Here's how the part is built. I have some questions about the finished solid (model axes, mm). Face numbers are marked on the shaded views. Round coordinates to 2 decimals unless told otherwise and drop trailing zeros. Loops run counter-clockwise (first coordinate to the right, second up) from the corner with the lowest first, then second, coordinate; pieces in that order, holes last. Notation, with made-up numbers: (22, 39) - (51, 39) arc R18 ccw to (51, 74) - close; hole circle Ø5 at (-2.5, -1.5). An arc over 180 degrees is marked (long way). Answer as a JSON object with one key per item and string values. Group by question number.
1) I want a section at A-A, the plane x = 0. Please give me the cut outline in (y, z).
2) If we mould it in two halves opening along Y, with no side actions, what happens to the marked faces 1, 2 and 3? For each: pulls with the +Y half, pulls with the -Y half, needs draft (parallel to the pull), parting line crosses it, or undercut.
3) If I drill on line 1 along Z through (x, y) = (2, 3.5); line 2 along X through (y, z) = (34, 0.5); line 3 along Z through (x, y) = (-1, 4), over which ranges is the centre line in solid material (lowest first)? Write a range as [from, to].
4) Will these pins go through, and if not, where does the flat tip stop? P1, Ø2, axis at x = 3, y = 40.5, coming from the +Z side; P2, Ø1, axis at x = -1.5, z = -1.5, coming from the +Y side.
5) I want a section at B-B, the plane z = 0. Please give me the cut outline in (x, y), then the cut area to 3 significant figures.
6) I want a section at C-C, the plane y = 43. Please give me the cut outline in (x, z).
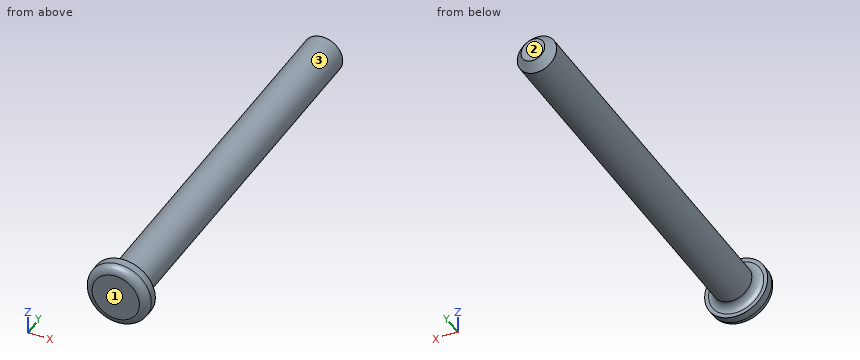
from build123d import *

# Parameters (mm, degrees)
SKETCH1_R           = 4
BOSS_EXTRUDE1_DEPTH = 2
SKETCH2_R           = 2.5
BOSS_EXTRUDE2_DEPTH = 50
FILLET1_R           = 1
CHAMFER1_SIZE       = 1
FILLET2_R           = 1


with BuildPart() as part:
    # Sketch1 → Boss-Extrude1 (new body)
    with BuildSketch(Plane(origin=(0, 0, 0), x_dir=(1, 0, 0), z_dir=(0, 1, 0))):
        with Locations(Location((0, 0, 0), (0, 0, 270))):
            Circle(SKETCH1_R)
    extrude(amount=BOSS_EXTRUDE1_DEPTH)

    # Sketch2 → Boss-Extrude2 (add)
    with BuildSketch(Plane(origin=(0, 2, 0), x_dir=(1, 0, 0), z_dir=(0, 1, 0))):
        with Locations(Location((0, 0, 0), (0, 0, 270))):
            Circle(SKETCH2_R)
    extrude(amount=BOSS_EXTRUDE2_DEPTH)

    # Fillet1
    fillet1_edges = [part.edges().sort_by_distance(p)[0] for p in [
        (0, 2, -2.5),
    ]]
    fillet(fillet1_edges, radius=FILLET1_R)

    # Chamfer1
    chamfer1_edges = [part.edges().sort_by_distance(p)[0] for p in [
        (0, 52, -2.5),
    ]]
    chamfer(chamfer1_edges, length=CHAMFER1_SIZE)

    # Fillet2
    fillet2_edges = [part.edges().sort_by_distance(p)[0] for p in [
        (0, 0, -4),
    ]]
    fillet(fillet2_edges, radius=FILLET2_R)


solid = part.part
Outcome:
{
 "1": {"outline": "(0, -3) arc R1 ccw to (1, -4) - (2, -4) - (2, -3.5) arc R1 cw to (3, -2.5) - (51, -2.5) - (52, -1.5) - (52, 1.5) - (51, 2.5) - (3, 2.5) arc R1 cw to (2, 3.5) - (2, 4) - (1, 4) arc R1 ccw to (0, 3) - close"},
 "2": {"face 1": "pulls with the -Y half", "face 2": "pulls with the +Y half", "face 3": "needs draft"},
 "3": {"line 1": "[-1.5, 1.5]", "line 2": "[-2.45, 2.45]", "line 3": "[-2.29, 2.29]"},
 "4": {"P1": "z = 1.5", "P2": "y = 51.88"},
 "5": {"outline": "(-4, 1) arc R1 ccw to (-3, 0) - (3, 0) arc R1 ccw to (4, 1) - (4, 2) - (3.5, 2) arc R1 cw to (2.5, 3) - (2.5, 51) - (1.5, 52) - (-1.5, 52) - (-2.5, 51) - (-2.5, 3) arc R1 cw to (-3.5, 2) - (-4, 2) - close", "area": "265 mm^2"},
 "6": {"outline": "circle Ø5 at (0, 0)"}
}
